Could you check a few things on this model? Use its own coordinates, in mm. A direction names the side the tool comes from. Coordinates: 2 decimals unless noted, no trailing zeros. Order: outer loops, then holes, each group sorted by start corner. A loop starts at its lowest first (then second) coordinate and runs counter-clockwise, first axis right, second up. Notation, with made-up numbers: (80, 42.25) -> (118, 42.25) arc R30 cw to (118, 70.25) -> close; hole circle Ø11 at (81, 76.5). An arc over 180 degrees is marked (long way). Use a Markdown table: item, result. Add a question column.
1) If we section it at B-B (y = 43): Write out the boundary of the cut face in (x, z), plus the area to 3 significant figures.
2) If we section it at A-A (x = 77.5): Write out the boundary of the cut face in (y, z), plus the area to 3 significant figures.
3) Which directions (+Z, -Z, +X, -X, +Y, -Y) give clear straight access to the entire face, cutting with the end or side of a thin tool? Please do faces 1 (the flat face through (25.4, 33, 32)), 2 (the flat face through (63.5, 33, 10)), 3 (the flat face through (34, 66.548, 18)).
4) If I drill on L1, parallel to Z at x = 57, y = 14; L2, parallel to X at y = 36, z = 23; L3, parallel to Y at x = 111, z = 13.5, over which ranges is the centre line in solid material (lowest first)? Write a range as [from, to].
5) If we section it at D-D (x = 100.5): Write out the boundary of the cut face in (y, z).
6) Thinking about a two-plate mould opening in Y: for faces 4 (the flat face through (105, 6.36, 9.66)), 5 (the flat face through (104.55, 60.21, 9.66)), 6 (the flat face through (0, 33, 23)), 7 (the flat face through (92, 40.835, 10)), which applies, +Y half, -Y half, draft (parallel to the pull), parting line (faces both ways), or undercut?
7) If we section it at C-C (z = 6.5): Write out the boundary of the cut face in (x, y), plus the area to 3 significant figures.
8) Will these pins go through, and if not, where does the flat tip stop? pin 1 Ø15 at (x, z) = (100, 12) entering from +Y; pin 2 Ø2 at (y, z) = (16, 25) entering from +X; pin 3 Ø6 at (x, y) = (41.5, 32.5) entering from +Z.
```python
from build123d import *

# Parameters (mm, degrees)
F1_DEPTH = 66.548
F2_W     = 57.15
F2_H     = 8.186824
F2_H_2   = 7.561176
F3_DEPTH = 19.051
F5_DEPTH = 19.051


with BuildPart() as f1:
    # F0 (on Front) → F1 (new body)
    with BuildSketch(Plane.XZ):
        Polygon((0, 44.45), (0, 0), (120.65, 0), (120.65, 19.05), (25.4, 19.05), (25.4, 44.45), align=None)
    extrude(amount=-F1_DEPTH)

    # F2 (on face) → F3 (cut, through all)
    with BuildSketch(Plane.XY.offset(19.05)):
        with Locations((92.075, 29.180588)):
            Rectangle(F2_W, F2_H)
        with Locations((92.075, 37.054588)):
            Rectangle(F2_W, F2_H_2)
    extrude(amount=-F3_DEPTH, mode=Mode.SUBTRACT)

    # F4 (on face) → F5 (cut, through all)
    with BuildSketch(Plane.XY.offset(19.05)):
        Polygon((88.9, 0), (120.65, 0), (120.65, 12.543588), align=None)
        Polygon((120.65, 53.691588), (120.65, 66.548), (88.9, 66.548), align=None)
    extrude(amount=-F5_DEPTH, mode=Mode.SUBTRACT)


solid = f1.part
```
Answer sheet:
| question | item | result |
|---|---|---|
| 1 | outline | (0, 0) -> (120.65, 0) -> (120.65, 19.05) -> (25.4, 19.05) -> (25.4, 44.45) -> (0, 44.45) -> close |
| 1 | area | 2,940 mm2 |
| 2 | outline | (0, 0) -> (25.09, 0) -> (25.09, 19.05) -> (0, 19.05) -> close; (40.84, 0) -> (66.55, 0) -> (66.55, 19.05) -> (40.84, 19.05) -> close |
| 2 | area | 968 mm2 |
| 3 | face 1 | +Z, +X, +Y, -Y |
| 3 | face 2 | +Z, -Z, +X |
| 3 | face 3 | +Z, -Z, +X, -X, +Y |
| 4 | L1 | [0, 19.05] |
| 4 | L2 | [0, 25.4] |
| 4 | L3 | [8.73, 25.09], [40.84, 57.6] |
| 5 | outline | (4.58, 0) -> (25.09, 0) -> (25.09, 19.05) -> (4.58, 19.05) -> close; (40.84, 0) -> (61.85, 0) -> (61.85, 19.05) -> (40.84, 19.05) -> close |
| 6 | face 4 | -Y half |
| 6 | face 5 | +Y half |
| 6 | face 6 | draft |
| 6 | face 7 | undercut |
| 7 | outline | (0, 0) -> (88.9, 0) -> (120.65, 12.54) -> (120.65, 25.09) -> (63.5, 25.09) -> (63.5, 40.84) -> (120.65, 40.84) -> (120.65, 53.69) -> (88.9, 66.55) -> (0, 66.55) -> close |
| 7 | area | 6,730 mm2 |
| 8 | pin 1 | y = 65.09 |
| 8 | pin 2 | x = 25.4 |
| 8 | pin 3 | z = 19.05 |
